Input: part model. Units: mm. Frame: model coordinates. Give positions to 0.01 mm unless a question says otherwise; leave off trailing zeros. Write each loop counter-clockwise with the first axis right and the second up, starting at its lowest first coordinate (ties: lowest second). Pieces come first, ordered by that corner, then holes. Notation, with made-up numbers: (73, -24) - (116, -24) arc R17 cw to (116, -3) - close; hole circle Ø11 at (54, 20). An arc over 180 degrees is marked (long way). Answer as CSV lines item,"result".
```python
from build123d import *

# Parameters (mm, degrees)
SKETCH002_W   = 435
SKETCH002_H   = 435
PAD_DEPTH     = 3
SKETCH001_R   = 2.25
SKETCH001_R_2 = 6.5
SKETCH001_R_3 = 11
SKETCH001_W   = 20
SKETCH001_H   = 20
POCKET_DEPTH  = 5


with BuildPart() as part:
    # Sketch002 → Pad (new body)
    with BuildSketch(Plane.XY):
        with Locations((217.5, 217.5)):
            Rectangle(SKETCH002_W, SKETCH002_H)
    extrude(amount=PAD_DEPTH)

    # Sketch001 → Pocket (cut)
    with BuildSketch(Plane.XY.offset(3)):
        with Locations((7.5, 31.5)):
            Circle(SKETCH001_R)
        with Locations((31.5, 7.5)):
            Circle(SKETCH001_R)
        with Locations((7.5, 403.5)):
            Circle(SKETCH001_R)
        with Locations((31.5, 427.5)):
            Circle(SKETCH001_R)
        with Locations((403.5, 427.5)):
            Circle(SKETCH001_R)
        with Locations((427.5, 403.5)):
            Circle(SKETCH001_R)
        with Locations((403.5, 7.5)):
            Circle(SKETCH001_R)
        with Locations((427.5, 31.5)):
            Circle(SKETCH001_R)
        with Locations((32.5, 62.5)):
            Circle(SKETCH001_R_2)
        with Locations((52.5, 39.5)):
            Circle(SKETCH001_R_3)
        with Locations((402.5, 62.5)):
            Circle(SKETCH001_R_2)
        with Locations((382.5, 39.5)):
            Circle(SKETCH001_R_3)
        with Locations((7.5, 7.5)):
            Rectangle(SKETCH001_W, SKETCH001_H)
        with Locations((427.5, 7.5)):
            Rectangle(SKETCH001_W, SKETCH001_H)
        with Locations((7.5, 427.5)):
            Rectangle(SKETCH001_W, SKETCH001_H)
        with Locations((427.5, 427.5)):
            Rectangle(SKETCH001_W, SKETCH001_H)
    extrude(amount=-POCKET_DEPTH, mode=Mode.SUBTRACT)


solid = part.part
```
Item 1: Cut plane B-B on x = 382.5. Return the cut outline in (y, z).
The answers:
outline,"(0, 0) - (28.5, 0) - (28.5, 3) - (0, 3) - close; (50.5, 0) - (435, 0) - (435, 3) - (50.5, 3) - close"
Item 2: Ray query, line 1 (Y direction, x = 403.5, z = 2.25); line 2 (Y direction, x = 7.5, z = 2.25); line 3 (X direction, y = 403.5, z = 1.8). Return the intervals inside material, ascending. Write a range as from..to.
The answers:
line 1,"0..5.25, 9.75..56.08, 68.92..425.25, 429.75..435"
line 2,"17.5..29.25, 33.75..401.25, 405.75..417.5"
line 3,"0..5.25, 9.75..425.25, 429.75..435"
Item 3: Contact query for flat-ended pins moving along their axis: pin 1 (0.9 mm diameter, centred on x = 11.5, z = 2, fed in from +Y); pin 2 (5 mm diameter, centred on x = 7.5, y = 403.5, fed in from -Z). Output: stop coordinate, or through.
The answers:
pin 1,"y = 417.5"
pin 2,"z = 0"
Item 4: Mould query, pull axis X, two halves, no side actions, for faces 1 (the face through (214, 221, 3)), 2 (the face through (408.5, 60, 1.5)). Classes: +X half, -X half, draft (parallel to the pull), parting line (faces both ways), or undercut.
The answers:
face 1,"draft"
face 2,"undercut"
Item 5: Cut plane A-A on y = 39.5. Return the cut outline in (x, z), plus the area to 3 significant figures.
The answers:
outline,"(0, 0) - (41.5, 0) - (41.5, 3) - (0, 3) - close; (63.5, 0) - (371.5, 0) - (371.5, 3) - (63.5, 3) - close; (393.5, 0) - (435, 0) - (435, 3) - (393.5, 3) - close"
area,"1,170 mm²"
